Can you work these out from the model? Positions are in its coordinate system, mm. A direction names the side the tool comes from. Give positions to 0.01 mm unless a question says otherwise; leave off trailing zeros.
Autodesk Inventor part; units mm, degrees
ref_plane "YZ Plane" through (0, 0, 0) normal (1, 0, 0) x (0, 1, 0)
ref_plane "XZ Plane" through (0, 0, 0) normal (0, 1, 0) x (-1, 0, 0)
ref_plane "XY Plane" through (0, 0, 0) normal (0, 0, 1) x (1, 0, 0)
sketch "Sketch1" plane through (0, 0, 0) normal (0, 1, 0) x (-1, 0, 0)
  line L0 (0, 0) -> (79, 0)
  line L1 (79, 0) -> (79, -56)
  line L2 (79, -56) -> (0, -56)
  line L3 (0, -56) -> (0, 0)
  dimension "d0" = 56
  dimension "d1" = 79
extrude "Extrusion1" add sketch "Sketch1" along normal blind 82
sketch "Sketch4" plane through (0, 0, 0) normal (0, -1, 0) x (1, 0, 0)
  line L0 (-78.5, -0.5) -> (-0.5, -0.5)
  line L1 (-0.5, -0.5) -> (-0.5, -55.5)
  line L2 (-0.5, -55.5) -> (-78.5, -55.5)
  line L3 (-78.5, -55.5) -> (-78.5, -0.5)
  line L4 (-78.5, -0.5) -> (-0.5, -55.5) construction
  line L5 (-0.5, -0.5) -> (-78.5, -55.5) construction
  line L6 (0, 0) -> (-79, 0)
  line L7 (-79, 0) -> (-79, -56)
  line L8 (-79, -56) -> (0, -56)
  line L9 (0, -56) -> (0, 0)
  point P0 (-39.5, -28)
  dimension "d4" = 0.5
  dimension "d5" = 0.5
  dimension "d7" = 0.5
  dimension "d8" = 0.5
extrude "Extrusion2" add sketch "Sketch4" along normal blind 1 contours L0 L1 L2 L3
sketch "Sketch5" plane through (0, -1, 0) normal (0, -1, 0) x (1, 0, 0)
  line L0 (-79, 0) -> (0, 0)
  line L1 (0, 0) -> (0, -56)
  line L2 (0, -56) -> (-79, -56)
  line L3 (-79, -56) -> (-79, 0)
  line L4 (-79, 0) -> (0, -56) construction
  line L5 (0, 0) -> (-79, -56) construction
  line L6 (0, -56) -> (0, 0)
  line L7 (-79, -56) -> (0, -56)
  line L8 (0, 0) -> (-79, 0)
  line L9 (-79, 0) -> (-79, -56)
  point P0 (-39.5, -28)
extrude "Extrusion3" add sketch "Sketch5" along normal blind 16
fillet "Fillet1" radius 2 4 edges at (-39.5, 82, -56) (0, 82, -28) (-39.5, 82, 0) (-79, 82, -28)
sketch "Sketch6" plane through (0, -17, 0) normal (0, -1, 0) x (1, 0, 0)
  line L0 (-11.5, -44.5) -> (-1.5, -44.5)
  line L1 (-1.5, -44.5) -> (-1.5, -54.5)
  line L2 (-1.5, -54.5) -> (-11.5, -54.5)
  line L3 (-11.5, -54.5) -> (-11.5, -44.5)
  line L4 (-11.5, -44.5) -> (-1.5, -54.5) construction
  line L5 (-1.5, -44.5) -> (-11.5, -54.5) construction
  line L6 (0, -56) -> (0, 0)
  line L7 (-79, -56) -> (0, -56)
  line L8 (-79, 0) -> (-79, -56)
  line L9 (-77.5, -44.5) -> (-67.5, -44.5)
  line L10 (-67.5, -44.5) -> (-67.5, -54.5)
  line L11 (-67.5, -54.5) -> (-77.5, -54.5)
  line L12 (-77.5, -54.5) -> (-77.5, -44.5)
  line L13 (-77.5, -44.5) -> (-67.5, -54.5) construction
  line L14 (-67.5, -44.5) -> (-77.5, -54.5) construction
  point P0 (-6.5, -49.5)
  point P1 (-72.5, -49.5)
  dimension "d14" = 10
  dimension "d15" = 10
  dimension "d16" = 1.5
  dimension "d17" = 1.5
  dimension "d18" = 10
  dimension "d19" = 10
  dimension "d20" = 1.5
  dimension "d21" = 1.5
extrude "Extrusion4" cut sketch "Sketch6" against normal blind 0.5
fillet "Fillet2" radius 0.5 4 edges at (-72.5, -16.5, -44.5) (-77.5, -16.5, -49.5) (-72.5, -16.5, -54.5) (-67.5, -16.5, -49.5)
fillet "Fillet3" radius 0.5 4 edges at (-11.5, -16.5, -49.5) (-6.5, -16.5, -44.5) (-6.5, -16.5, -54.5) (-1.5, -16.5, -49.5)
properties part number "battery" material "ABS Plastic"
1) For pin 1 Ø0.5 at (x, y) = (-45.5, -0.5) entering from +Z; pin 2 Ø0.8 at (y, z) = (-0.5, -39) entering from -X, each with a flat end and sliding along its axis, tell me the tip position at first contact or that it passes through.
Values follow:
pin 1: stops at z = -0.5
pin 2: stops at x = -78.5
2) If we mould it in two halves opening along Z, with no side actions, what happens to faces 3 (the face through (-40, 39, -56)), 4 (the face through (-7, -16.5, -49)), 5 (the face through (-40, -17, -28))? For each: +Z half, -Z half, draft (parallel to the pull), parting line (faces both ways), or undercut.
Values follow:
face 3: -Z half
face 4: undercut
face 5: draft
3) For faces 1 (the face through (-39, 39, 0)), 2 (the face through (-73, -16.5, -49)), which set-ups out of +Z, -Z, +X, -X, +Y, -Y let a thin tool reach every point of the face, with its end or its side?
Values follow:
face 1: +Z, +X, -X, +Y, -Y
face 2: -Y
4) Please list where this line runs through material, in increasing order: L1, parallel to Y at x = -9.5, z = -52.5.
Values follow:
L1: y = -16.5 to 82
